```python
from build123d import *

# Parameters (mm, degrees)
SKETCH_1_R               = 30
EXTRUDE_1_DEPTH          = 40
EXTRUDE_2_DEPTH          = 18
EXTRUDE_2_DEPTH_BACK     = 18
SKETCH_2_R               = 13.5
SKETCH_2_R_2             = 7.5
CUT_EXTRUDE_1_DEPTH      = 59.309518948
CUT_EXTRUDE_1_DEPTH_BACK = 59.309518948
SKETCH_3_W               = 20
SKETCH_3_H               = 17


with BuildPart() as part:
    # Sketch 1 → Extrude 1 (new body)
    with BuildSketch(Plane(origin=(0, 0, 0), x_dir=(0, 0, -1), z_dir=(1, 0, 0))):
        Circle(SKETCH_1_R)
    extrude(amount=EXTRUDE_1_DEPTH)

    # Sketch 2 → Extrude 2 (add, two sides: drawn at the far end of the back side and taken through both)
    # profile 1 of 2: a face of its own
    with BuildSketch(Plane(origin=(0, 0, 0), x_dir=(1, 0, 0), z_dir=(0, 1, 0)).offset(-EXTRUDE_2_DEPTH_BACK)):
        with BuildLine():
            Line((0, 13.5), (-15, 13.5))
            ThreePointArc((-15, 13.5), (-5.454058454, 9.545941546), (-1.5, 0))
            ThreePointArc((-1.5, 0), (-5.454058454, -9.545941546), (-15, -13.5))
            Line((-15, -13.5), (0, -13.5))
            Line((0, -13.5), (0, 13.5))
        make_face()
    # profile 2 of 2: a face of its own
    with BuildSketch(Plane(origin=(0, 0, 0), x_dir=(1, 0, 0), z_dir=(0, 1, 0)).offset(-EXTRUDE_2_DEPTH_BACK)):
        with Locations((-15, 0)):
            Circle(SKETCH_2_R)
        with Locations(Location((-15, 0, 0), (0, 0, 270))):
            Circle(SKETCH_2_R_2, mode=Mode.SUBTRACT)
    extrude(amount=EXTRUDE_2_DEPTH + EXTRUDE_2_DEPTH_BACK)

    # Sketch 3 → Cut-Extrude 1 (cut, two sides: drawn at the far end of the back side and taken through both)
    with BuildSketch(Plane.XY.offset(-CUT_EXTRUDE_1_DEPTH_BACK)):
        with Locations((10, 0)):
            Rectangle(SKETCH_3_W, SKETCH_3_H)
    extrude(amount=CUT_EXTRUDE_1_DEPTH + CUT_EXTRUDE_1_DEPTH_BACK, mode=Mode.SUBTRACT)


solid = part.part
```
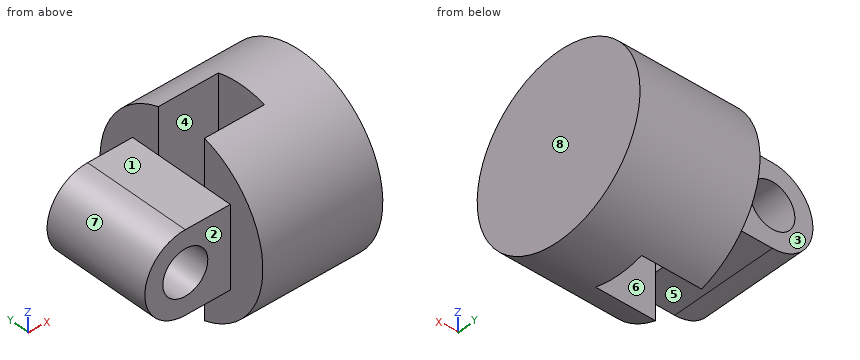
CAD build for the part. Positions are in the model's coordinates, mm. Face numbers are marked on the shaded views. A direction names the side the tool comes from. Give positions to 0.01 mm unless a question says otherwise; leave off trailing zeros. Loops run counter-clockwise (first coordinate to the right, second up) from the corner with the lowest first, then second, coordinate; pieces in that order, holes last. Notation, with made-up numbers: (10, 35.5) -> (45, 35.5) arc R17 cw to (45, 61.5) -> close; hole circle Ø1 at (79, -40). An arc over 180 degrees is marked (long way). Use a Markdown table: item, result.
1. Mould opens along X. For the marked faces 6, 7 and 8 say: pulls with the +X half, pulls with the -X half, needs draft (parallel to the pull), parting line crosses it, or undercut.
Check result:
| item | result |
|---|---|
| face 6 | undercut |
| face 7 | pulls with the -X half |
| face 8 | pulls with the +X half |
2. Slice it at D-D (z = -24). List the corners of the cut face in (x, y).
Check result:
| item | result |
|---|---|
| outline | (0, -18) -> (40, -18) -> (40, 18) -> (0, 18) -> (0, 8.5) -> (20, 8.5) -> (20, -8.5) -> (0, -8.5) -> close |
3. Slice it at A-A (y = 0). List the corners of the cut face in (x, z).
Check result:
| item | result |
|---|---|
| outline | (-15, -13.5) -> (0, -13.5) -> (0, 13.5) -> (-15, 13.5) arc R13.5 ccw to start; (20, -30) -> (40, -30) -> (40, 30) -> (20, 30) -> close; hole circle Ø15 at (-15, 0) |
4. Slice it at B-B (z = 0). List the corners of the cut face in (x, y), plus the area to 3 significant figures.
Check result:
| item | result |
|---|---|
| outline | (-28.5, -18) -> (-22.5, -18) -> (-22.5, 18) -> (-28.5, 18) -> close; (-7.5, -18) -> (0, -18) -> (0, -30) -> (40, -30) -> (40, 30) -> (0, 30) -> (0, 18) -> (-7.5, 18) -> close; hole (0, -8.5) -> (20, -8.5) -> (20, 8.5) -> (0, 8.5) -> close |
| area | 2,550 mm^2 |
5. Wall check: L1, parallel to X at y = 3, z = 0; L2, parallel to Y at x = -9, z = -7.5. Give the ranges that are in metal, low to high. Write a range as [from, to].
Check result:
| item | result |
|---|---|
| L1 | x = [-28.5, -22.5], [-7.5, 0], [20, 40] |
| L2 | y = [-18, 18] |
6. Which spindle directions (+Z, -Z, +X, -X, +Y, -Y) get a long thin tool onto all of the face, cutting with end or side? Do the marked faces 1, 2, 3, 4 and 5. Say none if no direction does.
Check result:
| item | result |
|---|---|
| face 1 | +Z, -X, +Y, -Y |
| face 2 | +Z, -Z, -X, -Y |
| face 3 | +Z, -Z, -X, +Y |
| face 4 | +Z, -Z |
| face 5 | -Z, -X, +Y, -Y |
7. Slice it at C-C (x = -9.5). List the corners of the cut face in (y, z), plus the area to 3 significant figures.
Check result:
| item | result |
|---|---|
| outline | (-18, -13.5) -> (18, -13.5) -> (18, -5.1) -> (-18, -5.1) -> close; (-18, 5.1) -> (18, 5.1) -> (18, 13.5) -> (-18, 13.5) -> close |
| area | 605 mm^2 |
8. Flat gauge pins, fed straight in: pin 1 (4 mm diameter, centred on y = -14.5, z = 22, fed in from -X); pin 2 (12 mm diameter, centred on x = 8, z = 11.5, fed in from +Y); pin 3 (12 mm diameter, centred on x = 0.5, z = 3, fed in from +Y); pin 4 (10 mm diameter, centred on x = 18.5, z = 14.5, fed in from +Y). Where does each tip first touch, or does it go through?
Check result:
| item | result |
|---|---|
| pin 1 | stops at x = 0 |
| pin 2 | stops at y = 29.49 |
| pin 3 | stops at y = 30 |
| pin 4 | stops at y = 28.46 |
